from build123d import *

# Parameters (mm, degrees)
SKETCH_R        = 7.95
PAD_DEPTH       = 5
SKETCH003_W     = 5
SKETCH003_H     = 2
SKETCH003_W_2   = 4
SKETCH003_H_2   = 3
POCKET_DEPTH    = 5.001
SKETCH002_W     = 5
SKETCH002_H     = 2
SKETCH002_W_2   = 4
SKETCH002_H_2   = 3
POCKET001_DEPTH = 5.001
POCKET002_DEPTH = 5.001


with BuildPart() as part:
    # Sketch → Pad (new body)
    with BuildSketch(Plane.XY):
        with BuildLine():
            add(Edge.make_bspline(
                [(-20, 150), (-20, 60), (-38.5, -100), (-90, -150)],
                knots=[0, 0, 0, 0, 1, 1, 1, 1], degree=3))
            Line((-20, 150), (-6, 150))
            Line((-6, 150), (-6, 175))
            Line((-6, 175), (6, 175))
            Line((6, 175), (6, 150))
            Line((6, 150), (20, 150))
            add(Edge.make_bspline(
                [(90, -150), (38.5, -100), (20, 60), (20, 150)],
                knots=[0, 0, 0, 0, 1, 1, 1, 1], degree=3))
            Line((90, -150), (90, -170))
            Line((90, -170), (-90, -170))
            Line((-90, -170), (-90, -150))
        make_face()
        with Locations((0, -100)):
            Circle(SKETCH_R, mode=Mode.SUBTRACT)
        with Locations((0, 100)):
            Circle(SKETCH_R, mode=Mode.SUBTRACT)
    extrude(amount=PAD_DEPTH)

    # Sketch003 (on Face28 of Pad) → Pocket (cut, through all)
    with BuildSketch(Plane(origin=(0, 100, 5), x_dir=(0, 1, 0), z_dir=(0, 0, 1))):
        with Locations((-25, 15)):
            Rectangle(SKETCH003_W, SKETCH003_H)
        with Locations((25, 15)):
            Rectangle(SKETCH003_W, SKETCH003_H)
        with Locations((25, -15)):
            Rectangle(SKETCH003_W, SKETCH003_H)
        with Locations((-25, -15)):
            Rectangle(SKETCH003_W, SKETCH003_H)
        with Locations((-29, 1.5)):
            Rectangle(SKETCH003_W_2, SKETCH003_H_2)
        with Locations((-21, 1.5)):
            Rectangle(SKETCH003_W_2, SKETCH003_H_2)
        with Locations((21, -1.5)):
            Rectangle(SKETCH003_W_2, SKETCH003_H_2)
        with Locations((29, -1.5)):
            Rectangle(SKETCH003_W_2, SKETCH003_H_2)
    extrude(amount=-POCKET_DEPTH, mode=Mode.SUBTRACT)

    # Sketch002 (on Face28 of Pad) → Pocket001 (cut, through all)
    with BuildSketch(Plane.XY.offset(5)):
        with Locations((-25, -85)):
            Rectangle(SKETCH002_W, SKETCH002_H)
        with Locations((25, -85)):
            Rectangle(SKETCH002_W, SKETCH002_H)
        with Locations((25, -115)):
            Rectangle(SKETCH002_W, SKETCH002_H)
        with Locations((-25, -115)):
            Rectangle(SKETCH002_W, SKETCH002_H)
        with Locations((21, -98.5)):
            Rectangle(SKETCH002_W_2, SKETCH002_H_2)
        with Locations((29, -98.5)):
            Rectangle(SKETCH002_W_2, SKETCH002_H_2)
        with Locations((-29, -101.5)):
            Rectangle(SKETCH002_W_2, SKETCH002_H_2)
        with Locations((-21, -101.5)):
            Rectangle(SKETCH002_W_2, SKETCH002_H_2)
    extrude(amount=-POCKET001_DEPTH, mode=Mode.SUBTRACT)

    # Sketch004 (on Face5 of Pocket001) → Pocket002 (cut, through all)
    with BuildSketch(Plane.XY.offset(5)):
        Polygon((-90, -150), (-80, -150), (-80, -170), (-60, -170), (-60, -150), (-45, -150), (-45, -170), (-25, -170), (-25, -150), (-10, -150), (-10, -170), (10, -170), (10, -150), (25, -150), (25, -170), (45, -170), (45, -150), (60, -150), (60, -170), (80, -170), (80, -150), (90, -150), (90, -180), (-90, -180), align=None)
    extrude(amount=-POCKET002_DEPTH, mode=Mode.SUBTRACT)


solid = part.part
CAD build for the part. Positions are in the model's coordinates, mm. Coordinates: 2 decimals unless noted, no trailing zeros. Write item = value, one per line. Start each with the question number.
Q1. Pull direction X, two halves, no side cores. Call faces 1 (the flat face through (-1, -33, 0)), 2 (the cylindrical face through (-1.035, -92.118, 2.465)): pulls with the +X half, pulls with the -X half, needs draft (parallel to the pull), parting line crosses it, or undercut.
Q2. Cut at A-A, the plane z = 1.5. Give the number of separate pieces and of enclosed holes in the cut face, then the cut area to 3 significant figures.
Q3. Flat gauge pins, fed straight in: pin 1 Ø2 at (x, z) = (15, 2.5) entering from -Y; pin 2 Ø2 at (x, z) = (15, 2.5) entering from +Y; pin 3 Ø2.5 at (y, z) = (-161, 1.5) entering from -X. Where does each tip first touch, or does it go through?
Q4. Drill centre lines: L1, parallel to Y at x = 1, z = 1.5; L2, parallel to X at y = 107, z = 0.8; L3, parallel to X at y = 78, z = 4. Where is each one in solid material? Low to high.
Computed:
q1.face_1 = needs draft
q1.face_2 = undercut
q2.separate_pieces = 1
q2.enclosed_holes = 18
q2.area = 25,200 mm²
q3.pin_1 = -150
q3.pin_2 = 150
q3.pin_3 = -80
q4.L1 = -170 to -107.89, -92.11 to 92.11, 107.89 to 119, 123 to 127, 131 to 175
q4.L2 = -21.21 to -3.77, 3.77 to 21.21
q4.L3 = -23.19 to -3, 0 to 23.19
